Source: CAD feature listing. Evaluate the final solid. Frame: model axes, mm. Face numbers are marked on the shaded views. A direction names the side the tool comes from. Give positions to 0.01 mm unless a question says otherwise; leave off trailing zeros. Write each loop counter-clockwise with the first axis right and the second up, starting at its lowest first coordinate (ties: lowest second). Pieces come first, ordered by that corner, then holes. Notation, with made-up numbers: (42.5, 56) -> (54.5, 56) arc R15 cw to (54.5, 61) -> close; hole circle Ø11 at (-22.75, 20). An arc over 180 degrees is marked (long way). Use one line per item in the form item = value. Start each with the question number.
(1) Cut plane D-D, the plane x = 1.25. Output: boundary loops of the cut face in (y, z), and give its area (3 significant figures).
(2) First-contact query: P1, Ø6, axis at x = 2.5, z = -1.5, coming from the +Y side. Flat tip, straight axial feed; report the tip coordinate or a pass-through.
(3) Draft query along X for the marked faces 1, 2 and 3. Return one class per face: pulls with the +X half, pulls with the -X half, needs draft (parallel to the pull), parting line crosses it, or undercut.
(4) Cut plane C-C, the plane y = 1.5. Output: boundary loops of the cut face in (x, z), and give its area (3 significant figures).
(5) Cut plane A-A, the plane z = -5.75. Output: boundary loops of the cut face in (x, y).
(6) Material intervals for line 1 along Y through (x, z) = (4.55, 5.2); line 2 along Z through (x, y) = (-5.25, 1.15); line 3 along X through (y, z) = (2.75, -7.5), sorted ascending. Write a range as from..to.
(7) Cut plane B-B, the plane z = 5.2. Output: boundary loops of the cut face in (x, y).
(8) Set-up query: the marked faces 4, 5 and 6. Return all of +Z, -Z, +X, -X, +Y, -Y with unobstructed straight access to the full face (end or side cutting, diameter ignored); none if empty.
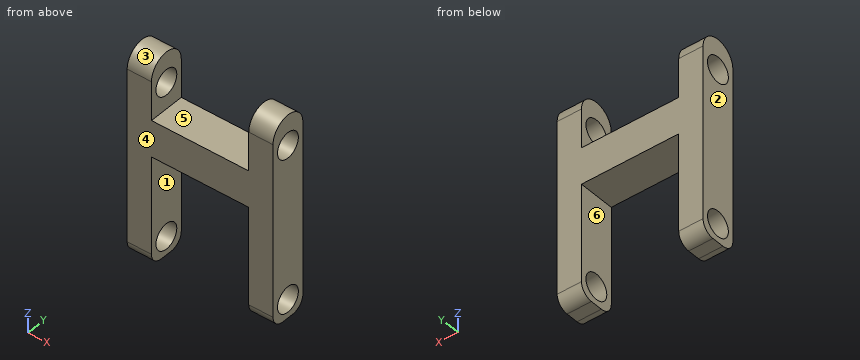
from build123d import *

# Parameters (mm, degrees)
EXTRUDE_1_DEPTH     = 3
SKETCH_2_OUTSIDE_W  = 13.724
SKETCH_2_OUTSIDE_H  = 8.024
CUT_EXTRUDE_1_DEPTH = 12
SKETCH_3_R          = 1.05
CUT_EXTRUDE_2_DEPTH = 12
FILLET_1_R          = 1
SKETCH_4_R          = 0.95
EXTRUDE_2_DEPTH     = 4
SKETCH_5_W          = 12
SKETCH_5_H          = 3
EXTRUDE_3_DEPTH     = 8
SKETCH_6_R          = 1.05
CUT_EXTRUDE_3_DEPTH = 12
CUT_EXTRUDE_4_DEPTH = 14.747727085
FILLET_2_R          = 1
SKETCH_9_W          = 11.8
SKETCH_9_H          = 3
EXTRUDE_4_DEPTH     = 4
SKETCH_10_W         = 8
SKETCH_10_H         = 4
CUT_EXTRUDE_5_DEPTH = 10
SKETCH_12_W         = 12
SKETCH_12_H         = 3
EXTRUDE_5_DEPTH     = 2
FILLET_3_R          = 1
SKETCH_13_W         = 12
SKETCH_13_H         = 2.969780185
CUT_EXTRUDE_6_DEPTH = 14.747727085
FILLET_4_R          = 1
SKETCH_15_W         = 8
SKETCH_15_H         = 4
CUT_EXTRUDE_7_DEPTH = 12.249216413
SKETCH_16_W         = 2
SKETCH_16_H         = 4.595961916
EXTRUDE_6_DEPTH     = 3


with BuildPart() as part:
    # 草图1 → 凸台-拉伸1 (new body)
    with BuildSketch(Plane(origin=(0, 0, 0), x_dir=(1, 0, 0), z_dir=(0, 1, 0))):
        Polygon((-6, 0), (6, 0), (6, -8.7), (4, -8.7), (4, -3), (-4, -3), (-4, -8.7), (-6, -8.7), align=None)
    extrude(amount=EXTRUDE_1_DEPTH)

    # 草图2 outside → 切除-拉伸1 (cut)
    with BuildSketch(Plane.ZY.offset(6)):
        with Locations((4.35, 1.5)):
            Rectangle(SKETCH_2_OUTSIDE_W, SKETCH_2_OUTSIDE_H)
        with BuildLine():
            Line((6.2, 3), (0, 3))
            Line((0, 3), (0, 0))
            Line((0, 0), (6.2, 0))
            ThreePointArc((6.2, 0), (7.7, 1.5), (6.2, 3))
        make_face(mode=Mode.SUBTRACT)
    extrude(amount=-CUT_EXTRUDE_1_DEPTH, mode=Mode.SUBTRACT)

    # 草图3 → 切除-拉伸2 (cut)
    with BuildSketch(Plane.ZY.offset(6)):
        with Locations((5.2, 1.5)):
            Circle(SKETCH_3_R)
    extrude(amount=-CUT_EXTRUDE_2_DEPTH, mode=Mode.SUBTRACT)

    # 圆角1
    fillet_1_edges = [part.edges().sort_by_distance(p)[0] for p in [
        (-6, 1.5, 0),
        (6, 1.5, 0),
    ]]
    fillet(fillet_1_edges, radius=FILLET_1_R)

    # 草图4 → 凸台-拉伸2 (add)
    with BuildSketch(Plane(origin=(0, 0, 0), x_dir=(-1, 0, 0), z_dir=(0, 0, -1))):
        with Locations(Location((0, 1.5, 0), (0, 0, 180))):
            Circle(SKETCH_4_R)
    extrude(amount=EXTRUDE_2_DEPTH)

    # 草图5 → 凸台-拉伸3 (add)
    with BuildSketch(Plane(origin=(0, 0, -4), x_dir=(-1, 0, 0), z_dir=(0, 0, -1))):
        with Locations((0, 1.5)):
            Rectangle(SKETCH_5_W, SKETCH_5_H)
    extrude(amount=EXTRUDE_3_DEPTH)

    # 草图6 → 切除-拉伸3 (cut)
    with BuildSketch(Plane(origin=(6, 0, 0), x_dir=(0, 0, -1), z_dir=(1, 0, 0))):
        with Locations((7.5, 1.5)):
            Circle(SKETCH_6_R)
    extrude(amount=-CUT_EXTRUDE_3_DEPTH, mode=Mode.SUBTRACT)

    # 草图8 → 切除-拉伸4 (cut, through all)
    with BuildSketch(Plane(origin=(0, 3, 0), x_dir=(1, 0, 0), z_dir=(0, 1, 0))):
        Polygon((-1.5, 8), (1.5, 8), (4, 8), (4, 12), (1.5, 12), (-1.5, 12), (-4, 12), (-4, 8), align=None)
    extrude(amount=-CUT_EXTRUDE_4_DEPTH, mode=Mode.SUBTRACT)

    # 圆角2
    fillet_2_edges = [part.edges().sort_by_distance(p)[0] for p in [
        (-5, 0, -12),
        (5, 0, -12),
    ]]
    fillet(fillet_2_edges, radius=FILLET_2_R)

    # 草图9 → 凸台-拉伸4 (add)
    with BuildSketch(Plane.XY.offset(-4)):
        with Locations((0, 1.5)):
            Rectangle(SKETCH_9_W, SKETCH_9_H)
    extrude(amount=EXTRUDE_4_DEPTH)

    # 草图10 → 切除-拉伸5 (cut)
    with BuildSketch(Plane(origin=(0, 3, 0), x_dir=(1, 0, 0), z_dir=(0, 1, 0))):
        with Locations((0, 6)):
            Rectangle(SKETCH_10_W, SKETCH_10_H)
    extrude(amount=-CUT_EXTRUDE_5_DEPTH, mode=Mode.SUBTRACT)

    # 草图12 → 凸台-拉伸5 (add)
    with BuildSketch(Plane.XY.offset(-4)):
        with Locations((0, 1.5)):
            Rectangle(SKETCH_12_W, SKETCH_12_H)
    extrude(amount=EXTRUDE_5_DEPTH)

    # 圆角3
    # the kernel refuses this fillet: 1 mm, written as the material it takes off along each edge
    with BuildSketch(Plane(origin=(6, 4.089724736, -2), x_dir=(0, 0, -1), z_dir=(0, -1, 0)), Plane(origin=(-6, -1.089724736, -2), x_dir=(0, 0, -1), z_dir=(0, 1, 0))) as fillet_3_piece_1:
        with BuildLine():
            CenterArc((0.435889894, -1), FILLET_3_R, 90, 25.841932763)
            Line((0, -0.1), (-0.008717798, -0.082))
            ThreePointArc((-0.008717798, -0.082), (-0.02, -0.05), (-0.02, 0))
            Line((-0.02, 0), (0, 0.02))
            Line((0, 0.02), (0.435889894, 0.02))
            Line((0.435889894, 0.02), (0.435889894, 0))
        make_face()
    extrude(amount=5.179449472, mode=Mode.SUBTRACT)

    # 草图13 → 切除-拉伸6 (cut, through all)
    with BuildSketch(Plane.XZ):
        with Locations((0, -10.515109908)):
            Rectangle(SKETCH_13_W, SKETCH_13_H)
    extrude(amount=-CUT_EXTRUDE_6_DEPTH, mode=Mode.SUBTRACT)

    # 圆角4
    fillet_4_edges = [part.edges().sort_by_distance(p)[0] for p in [
        (5, 3, -9.030219815),
        (-5, 3, -9.030219815),
        (5, 0, -9.030219815),
        (-5, 0, -9.030219815),
    ]]
    fillet(fillet_4_edges, radius=FILLET_4_R)

    # 草图15 → 切除-拉伸7 (cut, through all)
    with BuildSketch(Plane.XZ):
        with Locations((0, -2)):
            Rectangle(SKETCH_15_W, SKETCH_15_H)
    extrude(amount=-CUT_EXTRUDE_7_DEPTH, mode=Mode.SUBTRACT)

    # 草图16 → 凸台-拉伸6 (add, through all)
    with BuildSketch(Plane.XZ):
        with Locations((-5, -0.242379669)):
            Rectangle(SKETCH_16_W, SKETCH_16_H)
        with Locations((5, -0.242379669)):
            Rectangle(SKETCH_16_W, SKETCH_16_H)
    extrude(amount=-EXTRUDE_6_DEPTH)


solid = part.part
Geometry says:
q1.outline = (0, 0) -> (3, 0) -> (3, 3) -> (0, 3) -> close
q1.area = 9.00 mm^2
q2.P1 = 3
q3.face_1 = undercut
q3.face_2 = pulls with the -X half
q3.face_3 = needs draft
q4.outline = (-6, -9.03) -> (-4, -9.03) -> (-4, -8.55) -> (-6, -8.55) -> close; (-6, -6.45) -> (-4, -6.45) -> (-4, 0) -> (4, 0) -> (4, -6.45) -> (6, -6.45) -> (6, 4.15) -> (4, 4.15) -> (4, 3) -> (-4, 3) -> (-4, 4.15) -> (-6, 4.15) -> close; (-6, 6.25) -> (-4, 6.25) -> (-4, 7.7) -> (-6, 7.7) -> close; (4, -9.03) -> (6, -9.03) -> (6, -8.55) -> (4, -8.55) -> close; (4, 6.25) -> (6, 6.25) -> (6, 7.7) -> (4, 7.7) -> close
q4.area = 74.1 mm^2
q5.outline = (-6, 0) -> (-4, 0) -> (-4, 3) -> (-6, 3) -> close; (4, 0) -> (6, 0) -> (6, 3) -> (4, 3) -> close
q6.line_1 = 0..0.45, 2.55..3
q6.line_2 = -9.03..-8.49, -6.51..4.21, 6.19..7.66
q6.line_3 = -6..-4, 4..6
q7.outline = (-6, 0) -> (-4, 0) -> (-4, 0.45) -> (-6, 0.45) -> close; (-6, 2.55) -> (-4, 2.55) -> (-4, 3) -> (-6, 3) -> close; (4, 0) -> (6, 0) -> (6, 0.45) -> (4, 0.45) -> close; (4, 2.55) -> (6, 2.55) -> (6, 3) -> (4, 3) -> close
q8.face_4 = +Z, -Z, +X, -X, -Y
q8.face_5 = +Z, +Y, -Y
q8.face_6 = -Z, +Y, -Y
